Input: part model. Units: mm. Frame: model coordinates. Give positions to 0.01 mm unless a question says otherwise; leave off trailing zeros. Loops run counter-clockwise (first coordinate to the right, second up) from the corner with the lowest first, then second, coordinate; pieces in that order, holes last. Notation, with made-up numbers: M -36.5,-33 L -6.5,-33 A18 ccw -6.5,-17 Z; hole C 15.25,62.5 d6. An arc over 180 degrees is marked long. One line per item, written item: value. Start each with the question number.
(1) Section A-A on x = 1. Output: boundary loops of the cut face in (y, z) (3 decimals), plus the area to 3 significant figures.
(2) Ray query, line 1 along Y through (x, z) = (-15, 1.65); line 2 along Y through (x, z) = (3, 0.6); line 3 along X through (y, z) = (-2, 2.15). Return the intervals inside material, ascending. Write a range as from..to.
(3) Section B-B on z = 2.5. Output: boundary loops of the cut face in (x, y).
```python
from build123d import *

# Parameters (mm, degrees)
F1_DEPTH = 3.175
F2_R     = 1.27
F3_R     = 1.27


with BuildPart() as f1:
    # F0 (on Top) → F1 (new body)
    with BuildSketch(Plane.XY):
        with BuildLine():
            ThreePointArc((30.4419, 13.208), (29.697951, 15.004051), (27.9019, 15.748))
            Line((27.9019, 15.748), (-27.9019, 15.748))
            ThreePointArc((-27.9019, 15.748), (-29.697951, 15.004051), (-30.4419, 13.208))
            Line((-30.4419, 13.208), (-30.4419, -13.208))
            ThreePointArc((-30.4419, -13.208), (-29.697951, -15.004051), (-27.9019, -15.748))
            Line((-27.9019, -15.748), (27.9019, -15.748))
            ThreePointArc((27.9019, -15.748), (29.697951, -15.004051), (30.4419, -13.208))
            Line((30.4419, -13.208), (30.4419, 13.208))
        make_face()
        with BuildLine():
            ThreePointArc((28.1305, -0.762), (25.601074, -6.868574), (19.4945, -9.398))
            Line((19.4945, -9.398), (-19.4945, -9.398))
            ThreePointArc((-19.4945, -9.398), (-25.601074, -6.868574), (-28.1305, -0.762))
            Line((-28.1305, -0.762), (-28.1305, 0.762))
            ThreePointArc((-28.1305, 0.762), (-25.601074, 6.868574), (-19.4945, 9.398))
            Line((-19.4945, 9.398), (19.4945, 9.398))
            ThreePointArc((19.4945, 9.398), (25.601074, 6.868574), (28.1305, 0.762))
            Line((28.1305, 0.762), (28.1305, -0.762))
        make_face(mode=Mode.SUBTRACT)
    extrude(amount=F1_DEPTH)

    # F2
    f2_edges = [f1.edges().sort_by_distance(p)[0] for p in [
        (0, -9.398, 3.175),
    ]]
    fillet(f2_edges, radius=F2_R)

    # F3
    f3_edges = [f1.edges().sort_by_distance(p)[0] for p in [
        (0, -9.398, 0),
        (25.601074, -6.868574, 0),
        (-25.601074, -6.868574, 0),
        (-25.601074, 6.868574, 0),
        (0, 9.398, 0),
        (25.601074, 6.868574, 0),
        (28.1305, 0, 0),
        (-28.1305, 0, 0),
    ]]
    fillet(f3_edges, radius=F3_R)


solid = f1.part
```
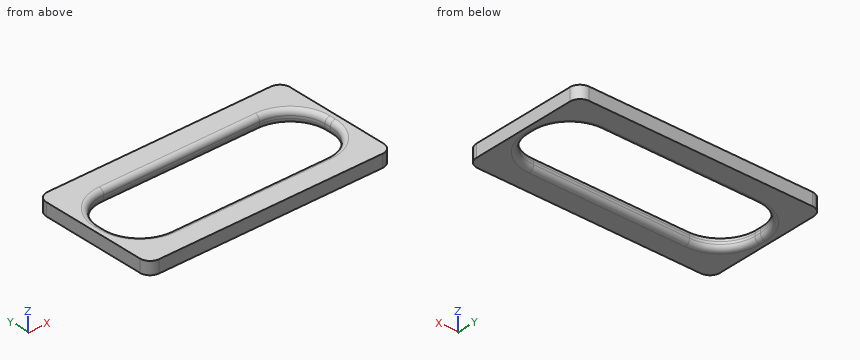
Output values:
1. outline: M -15.748,0 L -10.668,0 A1.27 ccw -9.398,1.27 L -9.398,1.905 A1.27 ccw -10.668,3.175 L -15.748,3.175 Z; M 9.398,1.27 A1.27 ccw 10.668,0 L 15.748,0 L 15.748,3.175 L 10.668,3.175 A1.27 ccw 9.398,1.905 Z
1. area: 38.9 mm²
2. line 1: y = -15.75..-9.4, 9.4..15.75
2. line 2: y = -15.75..-9.59, 9.59..15.75
2. line 3: x = -30.44..-28.07, 28.07..30.44
3. outline: M -30.44,-13.21 A2.54 ccw -27.9,-15.75 L 27.9,-15.75 A2.54 ccw 30.44,-13.21 L 30.44,13.21 A2.54 ccw 27.9,15.75 L -27.9,15.75 A2.54 ccw -30.44,13.21 Z; hole M -28.28,-0.76 A8.78 ccw -19.49,-9.55 L 19.49,-9.55 A8.78 ccw 28.28,-0.76 L 28.28,0.76 A8.78 ccw 19.49,9.55 L -19.49,9.55 A8.78 ccw -28.28,0.76 Z
